Autodesk Inventor part; units mm, degrees
ref_plane "YZ Plane" through (0, 0, 0) normal (1, 0, 0) x (0, 1, 0)
ref_plane "XZ Plane" through (0, 0, 0) normal (0, 1, 0) x (-1, 0, 0)
ref_plane "XY Plane" through (0, 0, 0) normal (0, 0, 1) x (1, 0, 0)
sketch "Sketch1" plane through (0, 0, 0) normal (0, 0, 1) x (1, 0, 0)
  arc A0 (251, 0) -> (0, 251) centre (0, 0) ccw
  arc A1 (0, 300) -> (300, 0) centre (0, 0) ccw construction
  circle A2 centre (0, 0) radius 320 construction
  line L0 (0, 0) -> (0, 251) construction
  line L1 (0, 0) -> (251, 0) construction
  arc A3 (300, 0) -> (0, 300) centre (0, 0) ccw
  line L2 (0, 251) -> (0, 300)
  arc A4 (0, 251) -> (251, 0) centre (0, 0) ccw construction
  line L3 (251, 0) -> (300, 0)
  dimension "d0" = 502
  dimension "d1" = 600
  dimension "d2" = 640
extrude "Plate1" add sketch "Sketch1" against normal blind 4
sketch "Sketch3" plane through (0, 0, 0) normal (0, 0, 1) x (1, 0, 0)
  circle A0 centre (0, 0) radius 275 construction
  line L0 (0, 0) -> (0, 300) construction
  arc A1 (300, 0) -> (0, 300) centre (0, 0) ccw
  line L1 (0, 0) -> (39.1579, 297.4335) construction
  circle A2 centre (35.8947, 272.6473) radius 8.5
  dimension "d12" = 550
  dimension "d13" = 7.5
  dimension "d14" = 17
extrude "Extrusion2" cut sketch "Sketch3" against normal through all
pattern_circular "Circular Pattern1" count 6 over 75 about axis through (0, 0, -10) along (0, 0, -1) of "Extrusion2"
equation "\"d5\" = Thickness"
equation "\"BendReliefWidth\" = Thickness"
equation "\"BendReliefDepth\" = 0.5 * Thickness"
equation "\"CornerReliefSize\" = 4 * Thickness"
equation "\"MinimumRemnant\" = 2 * Thickness"
equation "\"TransitionRadius\" = BendRadius"
equation "\"JacobiRadiusSize\" = BendRadius"
equation "\"GapSize\" = Thickness"
properties part number "MSC 403 FLANGE 500" material "Stainless Steel"
Design review of the part built by this model. Coordinates are the model's own, in mm. Give positions to 0.01 mm unless a question says otherwise; leave off trailing zeros. Loops run counter-clockwise (first coordinate to the right, second up) from the corner with the lowest first, then second, coordinate; pieces in that order, holes last. Notation, with made-up numbers: M 52,0 L 75,0 A24 ccw 75,32 Z; hole C 16.25,19 d10. An arc over 180 degrees is marked long. Answer as a JSON object with one key per item and string values.
Item 1: Mouldability with a two-part tool opening along Y and no side actions: class faces 1 (the face through (172, 184, -4)), 2 (the face through (34.05, 264.35, -1.97)), 3 (the face through (214.45, 209.79, -1.97)), 4 (the face through (172.581, 211.427, -1.972)) as pulls with the +Y half, pulls with the -Y half, needs draft (parallel to the pull), parting line crosses it, or undercut.
Output values:
{"face 1": "needs draft", "face 2": "undercut", "face 3": "pulls with the +Y half", "face 4": "undercut"}
Item 2: We need section B-B (x = 214). State the section outline as (y, z) points (3 decimals), and give its area (3 significant figures).
Output values:
{"outline": "M 131.168,-4 L 160.004,-4 L 160.004,0 L 131.168,0 Z; M 174.815,-4 L 210.247,-4 L 210.247,0 L 174.815,0 Z", "area": "257 mm2"}
Item 3: Wall thickness on line 1 along Y through (x, z) = (274.5, -0.35); line 2 along Y through (x, z) = (165, -0.65); line 3 along X through (y, z) = (112, -0.4): over which ranges is each line inside the solid? List them lowest first.
Output values:
{"line 1": "y = 0 to 27.6, 44.19 to 121.04", "line 2": "y = 189.15 to 210.02, 226.32 to 250.55", "line 3": "x = 224.63 to 248.92, 259.22 to 278.31"}
Item 4: We need section C-C (y = 222). State the section outline as (x, z) points.
Output values:
{"outline": "M 117.12,-4 L 159.82,-4 L 159.82,0 L 117.12,0 Z; M 175,-4 L 201.78,-4 L 201.78,0 L 175,0 Z"}
Item 5: We need section D-D (y = 151.5). State the section outline as (x, z) points, and give its area (3 significant figures).
Output values:
{"outline": "M 200.12,-4 L 258.94,-4 L 258.94,0 L 200.12,0 Z", "area": "235 mm2"}
